Check sheet for the modelled part. Datum: model origin and axes. Units: mm. Face numbers are marked on the shaded views. Round coordinates to 2 decimals unless told otherwise and drop trailing zeros. Loops run counter-clockwise (first coordinate to the right, second up) from the corner with the lowest first, then second, coordinate; pieces in that order, holes last. Notation, with made-up numbers: M 83.5,21 L 128.5,21 A19 cw 128.5,41 Z; hole C -34,47 d7. An arc over 180 degrees is marked long. Write item = value, one per line. Start each with the question number.
(1) Scan lines: L1, parallel to X at y = 4.25, z = 0; L2, parallel to Z at x = -0.25, y = 9.25; L3, parallel to Z at x = 2.25, y = 4.25. Record each from-to range of solid material in increasing order. Write a range as from..to.
(2) Cross-section at B-B on x = 0. Record the boundary of the cut face in (y, z), plus the area to 3 significant figures.
(3) Cross-section at D-D on z = 4.5. Record the boundary of the cut face in (x, y).
(4) Cross-section at C-C on x = -3.25. Record the boundary of the cut face in (y, z).
(5) Cross-section at A-A on z = 0. Record the boundary of the cut face in (x, y), plus the area to 3 significant figures.
(6) Mould release check, pull along X, two halves, no side actions. Record for the marked faces 1, 2 and 3: pulls with the +X half, pulls with the -X half, needs draft (parallel to the pull), parting line crosses it, or undercut.
(7) Go/stop test with flat-tipped pins: P1, Ø2, axis at x = -5.5, z = 9.5, coming from the -Y side; P2, Ø2, axis at x = 9, y = 8.5, coming from the +Z side; P3, Ø5, axis at x = 4.5, y = 5, coming from the -Z side; P4, Ø4, axis at x = -11, y = 2.5, coming from the -Z side. Record where each tip stops, or that it passes through.
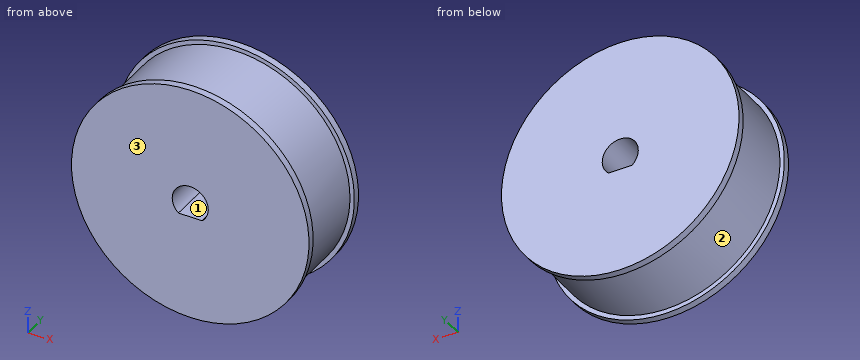
from build123d import *

# Parameters (mm, degrees)
BOSS_EXTRUDE1_START     = -9.6
BOSS_EXTRUDE1_DEPTH     = 9.6
CUT_EXTRUDE1_DEPTH      = 22.369604582
CUT_EXTRUDE1_DEPTH_BACK = 22.369604582


with BuildPart() as part:
    # Sketch1 → Revolve1 (revolve)
    with BuildSketch(Plane.XY, mode=Mode.PRIVATE) as revolve1_sk:
        Polygon((2, 0), (13.5, 0), (13.5, 0.8), (13, 0.8), (13, 8.8), (13.5, 8.8), (13.5, 9.6), (2, 9.6), align=None)
    revolve(revolve1_sk.sketch.rotate(Axis((0, 0, 0), (0, 1, 0)), 90), axis=Axis((0, 0, 0), (0, 1, 0)))

    # Sketch2 → Boss-Extrude1 (add)
    with BuildSketch(Plane(origin=(0, 9.6, 0), x_dir=(1, 0, 0), z_dir=(0, 1, 0)).offset(BOSS_EXTRUDE1_START)):
        with BuildLine():
            Line((-1.322875656, 1.5), (1.322875656, 1.5))
            ThreePointArc((1.322875656, 1.5), (0, 2), (-1.322875656, 1.5))
        make_face()
    extrude(amount=BOSS_EXTRUDE1_DEPTH)

    # Sketch4 → Cut-Extrude1 (cut, two sides: drawn at the far end of the back side and taken through both)
    with BuildSketch(Plane.XZ.offset(-CUT_EXTRUDE1_DEPTH_BACK)):
        with BuildLine():
            Line((-1.341640786, -1.55), (1.341640786, -1.55))
            ThreePointArc((1.341640786, -1.55), (0, 2.05), (-1.341640786, -1.55))
        make_face()
    extrude(amount=CUT_EXTRUDE1_DEPTH + CUT_EXTRUDE1_DEPTH_BACK, mode=Mode.SUBTRACT)


solid = part.part
Result:
q1.L1 = -13..-2.05, 2.05..13
q1.L2 = -13.5..-1.55, 2.03..13.5
q1.L3 = -12.8..12.8
q2.outline = M 0,-13.5 L 0.8,-13.5 L 0.8,-13 L 8.8,-13 L 8.8,-13.5 L 9.6,-13.5 L 9.6,-1.55 L 0,-1.55 Z; M 0,2.05 L 9.6,2.05 L 9.6,13.5 L 8.8,13.5 L 8.8,13 L 0.8,13 L 0.8,13.5 L 0,13.5 Z
q2.area = 217 mm^2
q3.outline = M -12.73,0 L 12.73,0 L 12.73,0.8 L 12.2,0.8 L 12.2,8.8 L 12.73,8.8 L 12.73,9.6 L -12.73,9.6 L -12.73,8.8 L -12.2,8.8 L -12.2,0.8 L -12.73,0.8 Z
q4.outline = M 0,-13.1 L 0.8,-13.1 L 0.8,-12.59 L 8.8,-12.59 L 8.8,-13.1 L 9.6,-13.1 L 9.6,13.1 L 8.8,13.1 L 8.8,12.59 L 0.8,12.59 L 0.8,13.1 L 0,13.1 Z
q5.outline = M -13.5,0 L -2.05,0 L -2.05,9.6 L -13.5,9.6 L -13.5,8.8 L -13,8.8 L -13,0.8 L -13.5,0.8 Z; M 2.05,0 L 13.5,0 L 13.5,0.8 L 13,0.8 L 13,8.8 L 13.5,8.8 L 13.5,9.6 L 2.05,9.6 Z
q5.area = 212 mm^2
q6.face_1 = undercut
q6.face_2 = parting line crosses it
q6.face_3 = needs draft
q7.P1 = 0
q7.P2 = 10.84
q7.P3 = -12.85
q7.P4 = -9.38
